Solid Edge part; units mm, degrees
sketch "Sketch1" plane through (0, 0, 0) normal (0, 0, 1) x (1, 0, 0)
  line L0 (-65, -65) -> (65, -65)
  line L1 (65, -65) -> (65, 65)
  line L2 (65, 65) -> (-65, 65)
  line L3 (-65, 65) -> (-65, -65)
extrude "Protrusion1" add sketch "Sketch1" along normal blind 130
shell "Thinwall1" thickness 3 removed faces 1 at (-44.6333, -42.0333, 0)
sketch "Sketch2" plane through (0, 0, 130) normal (0, 0, 1) x (1, 0, 0)
  line L0 (-35, 5) -> (-25, 5)
  line L1 (-25, 5) -> (-25, -5)
  line L2 (-25, -5) -> (-35, -5)
  line L3 (-35, -5) -> (-35, 5)
  line L4 (-20, 5) -> (-10, 5)
  line L5 (-10, 5) -> (-10, -5)
  line L6 (-10, -5) -> (-20, -5)
  line L7 (-20, -5) -> (-20, 5)
  circle A0 centre (-15, 15) radius 2.5
  circle A1 centre (-30, 15) radius 2.5
  circle A2 centre (0, 15) radius 2.5
  line L8 (-5, 5) -> (5, 5)
  line L9 (5, 5) -> (5, -5)
  line L10 (5, -5) -> (-5, -5)
  line L11 (-5, -5) -> (-5, 5)
  circle A3 centre (15, 15) radius 2.5
  line L12 (10, 5) -> (20, 5)
  line L13 (20, 5) -> (20, -5)
  line L14 (20, -5) -> (10, -5)
  line L15 (10, -5) -> (10, 5)
  circle A4 centre (30.6278, 15) radius 2.5
  line L16 (35.6278, 5) -> (25.6278, 5)
  line L17 (25.6278, 5) -> (25.6278, -5)
  line L18 (25.6278, -5) -> (35.6278, -5)
  line L19 (35.6278, -5) -> (35.6278, 5)
extrude "Cutout1" cut sketch "Sketch2" against normal up to next
Read the model definition and answer for the solid it produces. Units are mm, in the model's axes. A direction names the side the tool comes from. Give positions to 0.01 mm unless a question says otherwise; leave off trailing zeros. Loops run counter-clockwise (first coordinate to the right, second up) from the corner with the lowest first, then second, coordinate; pieces in that order, holes last.
Item 1: The part is cut by section A-A (x = -15). Write down the section's boundary in (y, z), and give its area (3 significant figures).
Item 2: The mould has two halves that part along Y. Classify faces 1 (the flat face through (-1, -14, 130)), 2 (the flat face through (-1, -65, 64)), 3 (the cylindrical face through (12.5, 15.1, 128.5)): released by +Y, released by -Y, zero draft, split by the parting line, or undercut.
Item 3: The part is cut by section D-D (y = -21.5). Write down the section's boundary in (x, z).
Item 4: The part is cut by section B-B (z = 35). Write down the section's boundary in (x, y).
Item 5: Each of these flat-tipped pins is pushed along its axis until it touches: pin 1 Ø8 at (x, y) = (0, 15) entering from -Z; pin 2 Ø4 at (x, y) = (30.63, 15) entering from +Z. Where does it stop, or does it pass through?
Item 6: The part is cut by section C-C (y = 15). Write down the section's boundary in (x, z).
Item 7: Find the intervals of material crossed by line 1 along Y through (x, z) = (15, 128.3); line 2 along X through (y, z) = (-51, 89), in increasing order.
Item 8: For faces 4 (the flat face through (65, -1, 64)), 5 (the flat face through (-1, -62, 63)), determine the directions among +Z, -Z, +X, -X, +Y, -Y from which every point of the face is accessible in a straight line to the end or side of a thin tool.
Taken from the geometry:
1. outline: (-65, 0) - (-62, 0) - (-62, 127) - (-5, 127) - (-5, 130) - (-65, 130) - close; (5, 127) - (12.5, 127) - (12.5, 130) - (5, 130) - close; (17.5, 127) - (62, 127) - (62, 0) - (65, 0) - (65, 130) - (17.5, 130) - close
1. area: 1,110 mm2
2. face 1: zero draft
2. face 2: released by -Y
2. face 3: undercut
3. outline: (-65, 0) - (-62, 0) - (-62, 127) - (62, 127) - (62, 0) - (65, 0) - (65, 130) - (-65, 130) - close
4. outline: (-65, -65) - (65, -65) - (65, 65) - (-65, 65) - close; hole (-62, -62) - (62, -62) - (62, 62) - (-62, 62) - close
5. pin 1: stops at z = 127
5. pin 2: passes through
6. outline: (-65, 0) - (-62, 0) - (-62, 127) - (-32.5, 127) - (-32.5, 130) - (-65, 130) - close; (-27.5, 127) - (-17.5, 127) - (-17.5, 130) - (-27.5, 130) - close; (-12.5, 127) - (-2.5, 127) - (-2.5, 130) - (-12.5, 130) - close; (2.5, 127) - (12.5, 127) - (12.5, 130) - (2.5, 130) - close; (17.5, 127) - (28.13, 127) - (28.13, 130) - (17.5, 130) - close; (33.13, 127) - (62, 127) - (62, 0) - (65, 0) - (65, 130) - (33.13, 130) - close
7. line 1: y = -65 to -5, 5 to 12.5, 17.5 to 65
7. line 2: x = -65 to -62, 62 to 65
8. face 4: +Z, -Z, +X, +Y, -Y
8. face 5: -Z
